Work out the finished part from the listing and answer in its coordinate system (mm). A direction names the side the tool comes from. Give positions to 0.01 mm unless a question says otherwise; leave off trailing zeros. Order: outer loops, then holes, each group sorted by start corner. A loop starts at its lowest first (then second) coordinate and runs counter-clockwise, first axis right, second up. Notation, with made-up numbers: (60, 10) -> (115, 10) arc R16 cw to (115, 36) -> close; hole circle Ø9 at (42.25, 24.5). An arc over 180 degrees is marked (long way). Answer as CSV lines item,"result". Start each with the question number.
1. A cutting plane is placed at A-A (y = 0). Give the vertices of the cut face in (x, z) (3 decimals), then the cut area to 3 significant figures.
2. For a pull along Y with two mould halves and no side action, classify faces 1 (the flat face through (3.131, -5.525, 2.862)), 2 (the flat face through (6.2, -2, 0)), 3 (the cylindrical face through (-7.559, 5.796, 0.939)) as released by +Y, released by -Y, zero draft, split by the parting line, or undercut.
3. A cutting plane is placed at B-B (z = -7). Give the vertices of the cut face in (x, y), then the cut area to 3 significant figures.
4. For faces 4 (the cylindrical face through (-1.38, -6.2, -17.22)), 5 (the flat face through (-2.5, 6.2, 3.175)), 6 (the flat face through (-3.219, -5.474, 2.862)), determine the directions among +Z, -Z, +X, -X, +Y, -Y from which every point of the face is accessible in a straight line to the end or side of a thin tool.
5. Flat-ended cylindrical pins translate along their axes: pin 1 (2 mm diameter, centred on y = 2.5, z = -25, fed in from -X); pin 2 (1.5 mm diameter, centred on y = 0.5, z = -27, fed in from -X); pin 3 (5 mm diameter, centred on x = 1.5, z = -27, fed in from -Y). Find the tip coordinate at first contact, or state that the pin passes through.
6. Find the intervals of material crossed by L1, parallel to Z at x = -5.25, y = 5.25 (3 decimals); L2, parallel to Y at x = 0, z = -11; L3, parallel to Z at x = -4.25, y = -2, in increasing order.
Solid Edge part; units mm, degrees
sketch "Sketch1" plane through (0, 0, 0) normal (0, 0, 1) x (1, 0, 0)
  circle A0 centre (0, 0) radius 6.35
extrude "Protrusion1" add sketch "Sketch1" against normal blind 38.1
sketch "Sketch2" plane through (0, 0, 0) normal (0, 0, 1) x (1, 0, 0)
  circle A0 centre (0, 0) radius 9.525
extrude "ExtrudedProtrusion_2" add sketch "Sketch2" along normal blind 3.175
sketch "Sketch3" plane through (0, 0, 3.175) normal (0, 0, 1) x (1, 0, 0)
  line L0 (0, 7.3323) -> (-6.35, 3.6662)
  line L1 (-6.35, 3.6662) -> (-6.35, -3.6662)
  line L2 (-6.35, -3.6662) -> (0, -7.3323)
  line L3 (0, -7.3323) -> (6.35, -3.6662)
  line L4 (6.35, -3.6662) -> (6.35, 3.6662)
  line L5 (6.35, 3.6662) -> (0, 7.3323)
extrude "ExtrudedCutout_1" cut sketch "Sketch3" against normal blind 0.635
chamfer "Chamfer_1" distance 3.175 angle 45 1 edges at (-6.35, 0, -38.1)
chamfer "Chamfer_2" distance 1.27 angle 45 1 edges at (-9.525, 0, 3.175)
Answer sheet:
1,outline,"(-9.525, 0) -> (-6.35, 0) -> (-6.35, -34.925) -> (-3.175, -38.1) -> (3.175, -38.1) -> (6.35, -34.925) -> (6.35, 0) -> (9.525, 0) -> (9.525, 1.905) -> (8.255, 3.175) -> (6.35, 3.175) -> (6.35, 2.54) -> (-6.35, 2.54) -> (-6.35, 3.175) -> (-8.255, 3.175) -> (-9.525, 1.905) -> close"
1,area,"525 mm^2"
2,face 1,"undercut"
2,face 2,"zero draft"
2,face 3,"split by the parting line"
3,outline,"circle Ø12.7 at (0, 0)"
3,area,"127 mm^2"
4,face 4,"-Z"
4,face 5,"+Z, +X, -X, +Y, -Y"
4,face 6,"+Z"
5,pin 1,"stops at x = -6.17"
5,pin 2,"stops at x = -6.35"
5,pin 3,"stops at y = -6.35"
6,L1,"z = 0 to 3.175"
6,L2,"y = -6.35 to 6.35"
6,L3,"z = -36.58 to 2.54"
